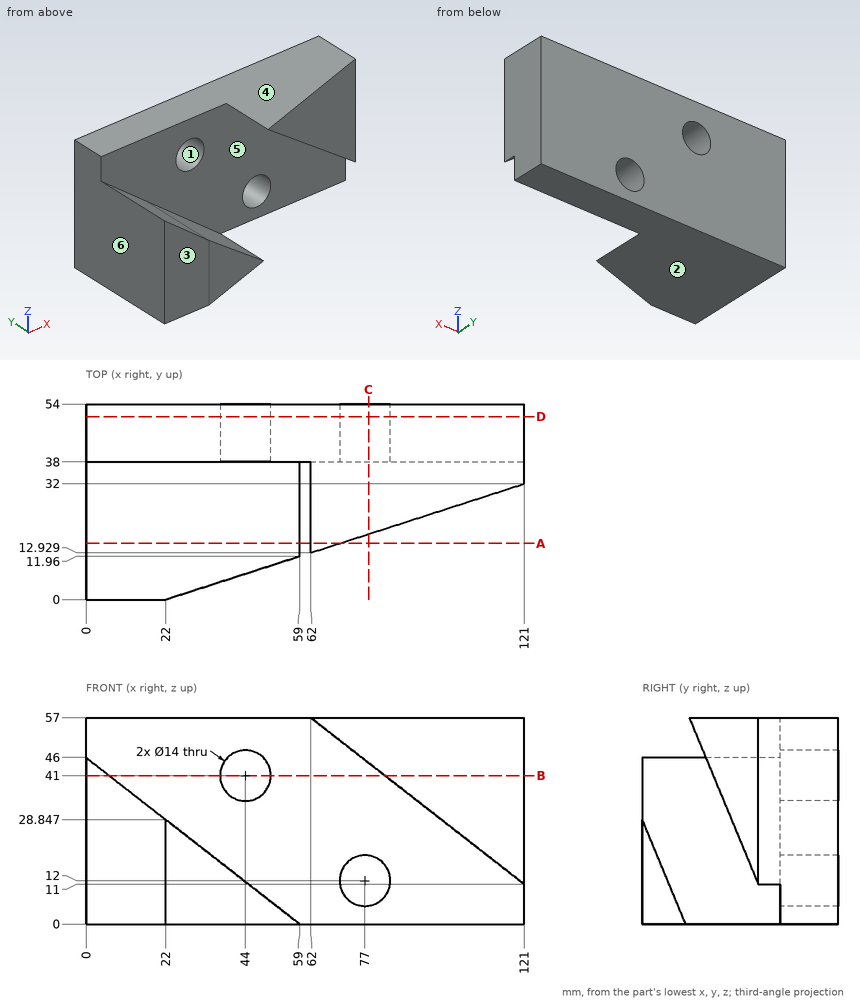
Design review of the part shown in the three views and the two pictorial views. Dimensions are in mm from the part's minimum x, y and z. A direction names the side the tool comes from. Round coordinates to 2 decimals unless told otherwise and drop trailing zeros. Write each loop counter-clockwise with the first axis right and the second up, starting at its lowest first coordinate (ties: lowest second). Pieces come first, ordered by that corner, then holes.
Item 1: The part is to be moulded in two halves that separate along Z. For the marked faces 1, 2, 3 and 4, say which applies: +Z half, -Z half, draft (parallel to the pull), parting line (faces both ways), or undercut.
Item 2: We need section C-C on x = 78. Write out the cut boundary in (y, z) (1 decimal).
Item 3: Clearance check with flat-ended pins moving along their axes: pin 1 Ø16 at (x, z) = (44, 41) entering from -Y; pin 2 Ø3 at (x, y) = (34.5, 16.5) entering from +Z; pin 3 Ø6 at (y, z) = (15.5, 15) entering from +X. State where each tip first meets the part, or that it passes through.
Item 4: For probe 1 along Z at (x, y) = (77, 42.25); probe 2 along Y at (x, z) = (93, 17); probe 3 along Z at (x, y) = (74, 44.5) (1 decimal), list the stretches that pass through material, from the lowest coordinate up.
Item 5: For the marked faces 5 and 6, list the 3-axis set-ups (+Z, -Z, +X, -X, +Y, -Y) from which the entire face can be reached by the end or side of a thin tool; tool diameter is ignored.
Item 6: We need section D-D on y = 50.5. Write out the cut boundary in (x, z).
Item 7: We need section A-A on y = 15.5. Write out the cut boundary in (x, z), and give its area (3 significant figures).
Item 8: We need section B-B on z = 41. Write out the cut boundary in (x, y).
Returned:
1. face 1: undercut
1. face 2: -Z half
1. face 3: draft
1. face 4: +Z half
2. outline: (18.1, 44.5) - (38, 44.5) - (38, 18.9) - (54, 18.9) - (54, 57) - (18.1, 57) - close; (38, 0) - (54, 0) - (54, 5.1) - (38, 5.1) - close
3. pin 1: stops at y = 38
3. pin 2: stops at z = 20.27
3. pin 3: stops at x = 43.61
4. probe 1: z = 0 to 5, 19 to 57
4. probe 2: y = 38 to 54
4. probe 3: z = 0 to 5.7, 18.3 to 57
5. face 5: -Y
5. face 6: +Z, -Z, -X, +Y, -Y
6. outline: (0, 0) - (121, 0) - (121, 57) - (0, 57) - close; hole circle Ø14 at (44, 41); hole circle Ø14 at (77, 12)
7. outline: (0, 0) - (59, 0) - (0, 46) - close; (62, 57) - (69.95, 50.8) - (69.95, 57) - close
7. area: 1,380 mm2
8. outline: (0, 0) - (6.41, 0) - (6.41, 38) - (37, 38) - (37, 54) - (0, 54) - close; (51, 38) - (82.52, 38) - (82.52, 19.56) - (121, 32) - (121, 54) - (51, 54) - close
